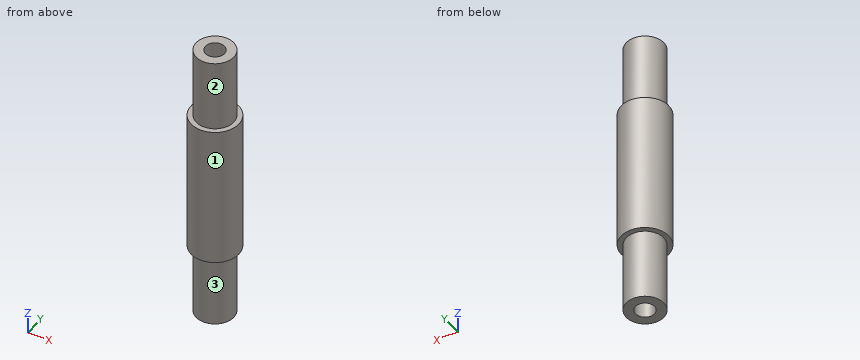
```python
from build123d import *

# Parameters (mm, degrees)
SKETCH1_R                  = 6.35
SKETCH1_R_2                = 5.0165
BOSS_EXTRUDE1_DEPTH        = 19.05
SKETCH1_4_R                = 5.0165
BOSS_EXTRUDE2_DEPTH        = 38.1
F_7_0_201_DIAMETER_HOLE1_D = 5.1054


with BuildPart() as part:
    # Sketch1 → Boss-Extrude1 (new, symmetric)
    with BuildSketch(Plane.XY):
        Circle(SKETCH1_R)
        Circle(SKETCH1_R_2, mode=Mode.SUBTRACT)
    extrude(amount=BOSS_EXTRUDE1_DEPTH, both=True)

    # Sketch1<4> → Boss-Extrude2 (add, symmetric)
    with BuildSketch(Plane.XY):
        Circle(SKETCH1_4_R)
    extrude(amount=BOSS_EXTRUDE2_DEPTH, both=True)

    # #7 (0.201) Diameter Hole1 (through all)
    with Locations(Plane(origin=(0, 0, -38.1), x_dir=(-1, 0, 0), z_dir=(0, 0, -1))):
        with Locations((0, 0)):
            Hole(F_7_0_201_DIAMETER_HOLE1_D / 2)


solid = part.part
```
Source: CAD feature listing. Evaluate the final solid. Frame: model axes, mm. Face numbers are marked on the shaded views. A direction names the side the tool comes from. Coordinates: 2 decimals unless noted, no trailing zeros. Order: outer loops, then holes, each group sorted by start corner. A loop starts at its lowest first (then second) coordinate and runs counter-clockwise, first axis right, second up. Notation, with made-up numbers: (-38, 38) - (3, 38) arc R10 ccw to (3, 53) - close; hole circle Ø2 at (78, -22). An arc over 180 degrees is marked (long way). One line per item, written item: value.
1) Ray query, line 1 (Y direction, x = 0, z = -17); line 2 (Z direction, x = 2.75, y = 4.75); line 3 (X direction, y = -1.5, z = -27). Return the intervals inside material, ascending. Write a range as [from, to].
Computed values:
line 1: y = [-6.35, -2.55], [2.55, 6.35]
line 2: z = [-19.05, 19.05]
line 3: x = [-4.79, -2.07], [2.07, 4.79]
2) Cut plane C-C on z = -23. Output: boundary loops of the cut face in (x, y), plus the area to 3 significant figures.
Computed values:
outline: circle Ø10.03 at (0, 0); hole circle Ø5.11 at (0, 0)
area: 58.6 mm^2
3) Cut plane A-A on x = 0. Output: boundary loops of the cut face in (y, z), plus the area to 3 significant figures.
Computed values:
outline: (-6.35, -19.05) - (-5.02, -19.05) - (-5.02, -38.1) - (-2.55, -38.1) - (-2.55, 38.1) - (-5.02, 38.1) - (-5.02, 19.05) - (-6.35, 19.05) - close; (2.55, -38.1) - (5.02, -38.1) - (5.02, -19.05) - (6.35, -19.05) - (6.35, 19.05) - (5.02, 19.05) - (5.02, 38.1) - (2.55, 38.1) - close
area: 477 mm^2
4) Contact query for a flat-ended pin moving along its axis: pin 1 (4 mm diameter, centred on x = -1, z = 28, fed in from +Y). Output: stop coordinate, or through.
Computed values:
pin 1: stops at y = 5.02
5) Reachability of the marked faces 1, 2 and 3 from +Z, -Z, +X, -X, +Y, -Y: full face, straight path, thin tool, end or side. Return the list, or none.
Computed values:
face 1: +Z, -Z
face 2: +Z
face 3: -Z
6) Cut plane D-D on x = 3.75. Output: boundary loops of the cut face in (y, z), plus the area to 3 significant figures.
Computed values:
outline: (-5.12, -19.05) - (-3.33, -19.05) - (-3.33, -38.1) - (3.33, -38.1) - (3.33, -19.05) - (5.12, -19.05) - (5.12, 19.05) - (3.33, 19.05) - (3.33, 38.1) - (-3.33, 38.1) - (-3.33, 19.05) - (-5.12, 19.05) - close
area: 644 mm^2
